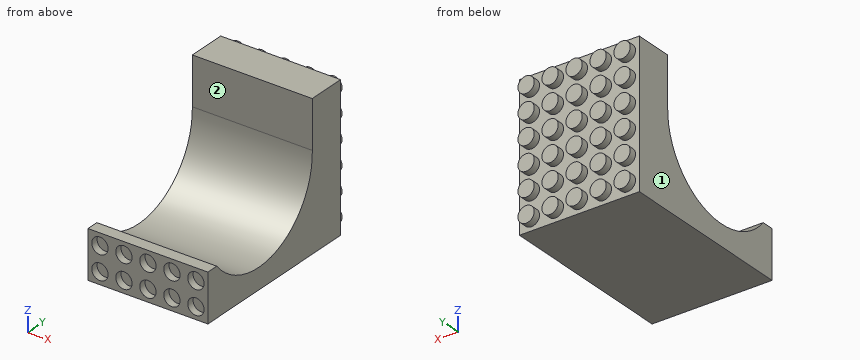
Autodesk Inventor part; units mm, degrees
ref_plane "YZ Plane" through (0, 0, 0) normal (1, 0, 0) x (0, 1, 0)
ref_plane "XZ Plane" through (0, 0, 0) normal (0, 1, 0) x (-1, 0, 0)
ref_plane "XY Plane" through (0, 0, 0) normal (0, 0, 1) x (1, 0, 0)
sketch "草圖1" plane through (0, 0, 0) normal (0, 1, 0) x (-1, 0, 0)
  line L0 (12.5, 12.5) -> (-12.5, 12.5)
  line L1 (-12.5, 12.5) -> (-12.5, -12.5)
  line L2 (-12.5, -12.5) -> (12.5, -12.5)
  line L3 (12.5, -12.5) -> (12.5, 12.5)
  circle A0 centre (10, 10) radius 1.7
  circle A1 centre (5, 10) radius 1.7
  circle A2 centre (0, 10) radius 1.7
  circle A3 centre (-5, 10) radius 1.7
  circle A4 centre (-10, 10) radius 1.7
  circle A5 centre (10, 5) radius 1.7
  circle A6 centre (5, 5) radius 1.7
  circle A7 centre (0, 5) radius 1.7
  circle A8 centre (-5, 5) radius 1.7
  circle A9 centre (-10, 5) radius 1.7
  circle A10 centre (10, 0) radius 1.7
  circle A11 centre (5, 0) radius 1.7
  circle A12 centre (0, 0) radius 1.7
  circle A13 centre (-5, 0) radius 1.7
  circle A14 centre (-10, 0) radius 1.7
  circle A15 centre (10, -5) radius 1.7
  circle A16 centre (5, -5) radius 1.7
  circle A17 centre (0, -5) radius 1.7
  circle A18 centre (-5, -5) radius 1.7
  circle A19 centre (-10, -5) radius 1.7
  circle A20 centre (10, -10) radius 1.7
  circle A21 centre (5, -10) radius 1.7
  circle A22 centre (0, -10) radius 1.7
  circle A23 centre (-5, -10) radius 1.7
  circle A24 centre (-10, -10) radius 1.7
  point P0 (0, 0)
  point P1 (12.5, 0)
  point P2 (0, -12.5)
  dimension "d0" = 25
  dimension "d1" = 25
  dimension "d10" = 3.4
  dimension "d11" = 2.5
  dimension "d12" = 2.5
  dimension "d15" = 5
  dimension "d18" = 5
sketch "草圖2" plane through (0, 0, 0) normal (1, 0, 0) x (0, 1, 0)
  line L0 (0, 12.5) -> (0, -12.5)
  line L1 (0, -12.5) -> (35, -12.5)
  line L2 (35, -12.5) -> (35, 12.5)
  line L3 (35, 12.5) -> (27, 12.5)
  line L4 (27, 12.5) -> (27, 7.5)
  line L5 (0, -12.5) -> (0, -2.5)
  arc A0 (0, -2.5) -> (27, 7.5) centre (11.8134, 7.0537) ccw
  point P0 (0, 0)
  dimension "d2" = 35
  dimension "d3" = 8
  dimension "d4" = 5
  dimension "d5" = 10
  dimension "d6" = 25
  dimension "d7" = 15.1931
extrude "擠出1" add sketch "草圖2" along normal mid plane 25
sketch "草圖3" plane through (-12.5, 35, 12.5) normal (0, 1, 0) x (1, 0, 0)
  circle A0 centre (22.5, 22.5) radius 1.7
  point P0 (12.5, 12.5)
extrude "擠出3" add sketch "草圖3" along normal blind 1.5
pattern_linear "矩形陣列1" count 5 spacing 5 along (-1, 0, 0) count 6 spacing 5 along (0, 0, 1) of "擠出3"
sketch "草圖4" plane through (-12.5, 27, 12.5) normal (0, 0, 1) x (1, 0, 0)
  line L0 (0, 0) -> (25, 0)
  line L1 (25, 8) -> (25, 0)
  line L2 (0, 8) -> (25, 8)
  line L3 (0, 0) -> (0, 8)
  line L4 (0, 8) -> (25, 8)
  line L5 (25, 8) -> (25, 0)
  line L6 (25, 0) -> (0, 0)
  line L7 (0, 0) -> (0, 8)
  point P0 (12.5, -27)
extrude "擠出4" add sketch "草圖4" along normal blind 5
sketch "草圖5" plane through (-12.5, 0, -12.5) normal (0, -1, 0) x (1, 0, 0)
  line L0 (0, 10) -> (25, 10)
  line L1 (25, 10) -> (25, 0)
  line L2 (0, 0) -> (25, 0)
  line L3 (0, 0) -> (0, 10)
  point P0 (12.5, 12.5)
extrude "擠出5" add sketch "草圖5" along normal blind 2.5
sketch "草圖6" plane through (-12.5, -2.5, -12.5) normal (0, -1, 0) x (1, 0, 0)
  circle A0 centre (22.5, 7.5) radius 1.7
  circle A1 centre (22.5, 2.5) radius 1.7
  circle A2 centre (17.5, 7.5) radius 1.7
  line L0 (25, 0) -> (25, 10)
  line L1 (25, 10) -> (0, 10)
  line L2 (0, 10) -> (0, 0)
  line L3 (0, 0) -> (25, 0)
  circle A3 centre (12.5, 7.5) radius 1.7
  circle A4 centre (12.5, 2.5) radius 1.7
  circle A5 centre (17.5, 2.5) radius 1.7
  circle A6 centre (7.5, 7.5) radius 1.7
  circle A7 centre (7.5, 2.5) radius 1.7
  circle A8 centre (2.5, 7.5) radius 1.7
  circle A9 centre (2.5, 2.5) radius 1.7
  point P0 (12.5, 12.5)
extrude "擠出6" cut sketch "草圖6" against normal blind 1.5 contours A0 | A1 | A2 | A3 | A4 | A5 | A6 | A7 | A8 | A9
properties part number "110033226_ipt_19_大橋接通道路"
Here's how the part is built. I have some questions about the finished solid (model axes, mm). Face numbers are marked on the shaded views. A direction names the side the tool comes from. Round coordinates to 2 decimals unless told otherwise and drop trailing zeros. Order: outer loops, then holes, each group sorted by start corner. A loop starts at its lowest first (then second) coordinate and runs counter-clockwise, first axis right, second up. Notation, with made-up numbers: (69.25, 37) -> (94.25, 37) arc R20 cw to (94.25, 70) -> close; hole circle Ø5 at (-1, 50). An arc over 180 degrees is marked (long way). Use CSV: the item, a comma, the result in double quotes.
1. Which directions (+Z, -Z, +X, -X, +Y, -Y) give clear straight access to the entire face, cutting with the end or side of a thin tool? Please do the marked faces 1 and 2.
Recorded:
face 1,"+Z, -Z, -X, +Y, -Y"
face 2,"+Z, +X, -X, -Y"
2. I'm going to push flat-ended pins straight in: P1, Ø1, axis at x = 0, z = -10.5, coming from the -Y side; P2, Ø10, axis at y = 18, z = 0.5, coming from the +X side; P3, Ø11, axis at x = 1, z = 15, coming from the -Y side. Where does each tip first touch, or does it pass through?
Recorded:
P1,"stops at y = -1"
P2,"passes through"
P3,"stops at y = 27"
3. I want a section at C-C on z = 0. List the corners of the cut face in (x, y) for me.
Recorded:
outline,"(-12.5, 25.27) -> (12.5, 25.27) -> (12.5, 35) -> (11.7, 35) -> (11.7, 36.5) -> (8.3, 36.5) -> (8.3, 35) -> (6.7, 35) -> (6.7, 36.5) -> (3.3, 36.5) -> (3.3, 35) -> (1.7, 35) -> (1.7, 36.5) -> (-1.7, 36.5) -> (-1.7, 35) -> (-3.3, 35) -> (-3.3, 36.5) -> (-6.7, 36.5) -> (-6.7, 35) -> (-8.3, 35) -> (-8.3, 36.5) -> (-11.7, 36.5) -> (-11.7, 35) -> (-12.5, 35) -> close"
4. I want a section at D-D on y = 14.5. List the corners of the cut face in (x, z) for me.
Recorded:
outline,"(-12.5, -12.5) -> (12.5, -12.5) -> (12.5, -7.9) -> (-12.5, -7.9) -> close"
5. I need wall thicknesses on line 1 along Z through (x, y) = (-10, -1.35); line 2 along Y through (x, z) = (-8, -6.5); line 3 along Y through (x, z) = (10, 7.5). Which ranges of each line are inside material? Lowest first, please.
Recorded:
line 1,"z = -12.5 to -11.7, -8.3 to -6.7, -3.3 to -2.5"
line 2,"y = -2.5 to 4.95, 18.68 to 35"
line 3,"y = 27 to 35"
6. I want a section at A-A on z = 15. List the corners of the cut face in (x, y) for me, and give its area (4 significant figures).
Recorded:
outline,"(-12.5, 27) -> (12.5, 27) -> (12.5, 35) -> (11.7, 35) -> (11.7, 36.5) -> (8.3, 36.5) -> (8.3, 35) -> (6.7, 35) -> (6.7, 36.5) -> (3.3, 36.5) -> (3.3, 35) -> (1.7, 35) -> (1.7, 36.5) -> (-1.7, 36.5) -> (-1.7, 35) -> (-3.3, 35) -> (-3.3, 36.5) -> (-6.7, 36.5) -> (-6.7, 35) -> (-8.3, 35) -> (-8.3, 36.5) -> (-11.7, 36.5) -> (-11.7, 35) -> (-12.5, 35) -> close"
area,"225.5 mm2"
7. I want a section at B-B on y = 10. List the corners of the cut face in (x, z) for me, and give its area (3 significant figures).
Recorded:
outline,"(-12.5, -12.5) -> (12.5, -12.5) -> (12.5, -8.03) -> (-12.5, -8.03) -> close"
area,"112 mm2"
